Geometry check sheet. Reference: drawing and pictorial views, mm from the part's lowest x, y, z. A direction names the side the tool comes from. Coordinates: 2 decimals unless noted, no trailing zeros. Loops run counter-clockwise (first coordinate to the right, second up) from the corner with the lowest first, then second, coordinate; pieces in that order, holes last.
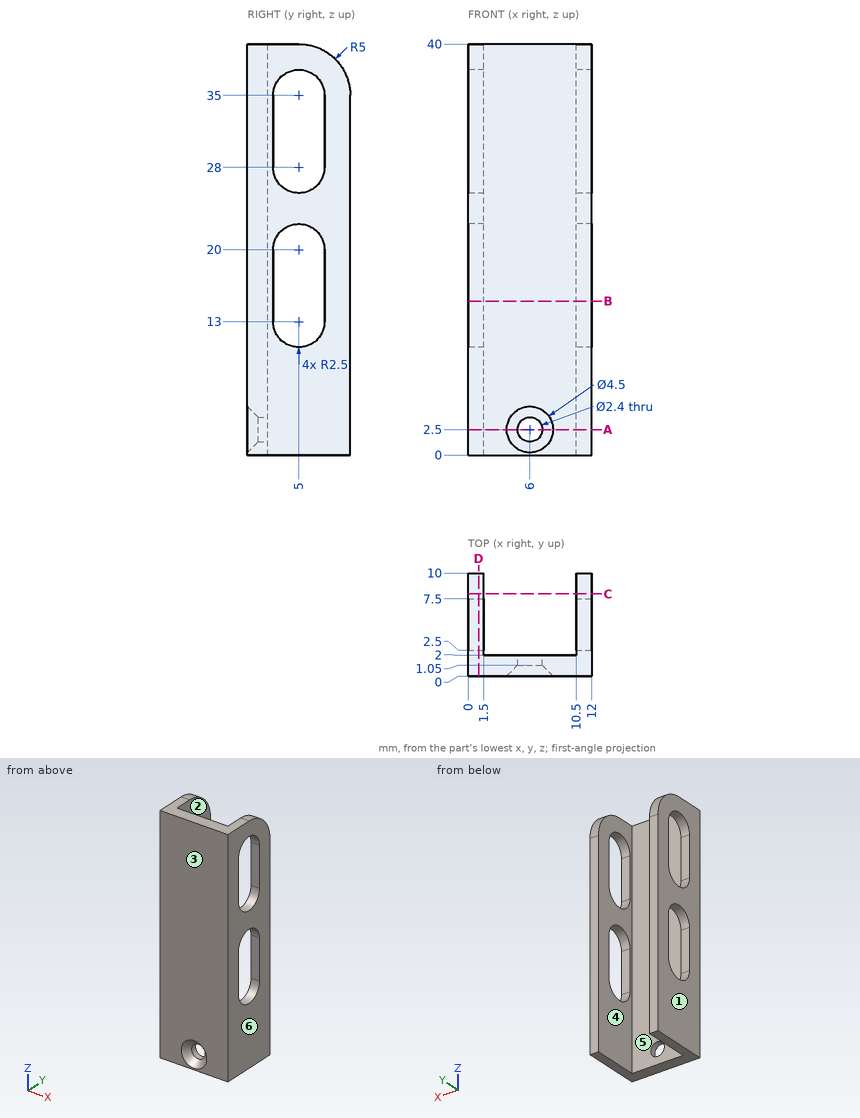
1) Depth check by flat-ended pin: pin 1 (1.2 mm diameter, centred on x = 0.5, z = 33, fed in from -Y); pin 2 (4 mm diameter, centred on x = 6, z = 2.5, fed in from +Y); pin 3 (4 mm diameter, centred on x = 8, y = 6.5, fed in from +Z). Enter the tip coordinate at first touch or a pass-through.
Data:
pin 1: stops at y = 0
pin 2: stops at y = 2
pin 3: passes through
2) Section check C-C on y = 8. Record the cut outline in (x, z).
Data:
outline: (0, 0) - (1.5, 0) - (1.5, 39) - (0, 39) - close; (10.5, 0) - (12, 0) - (12, 39) - (10.5, 39) - close
3) Section check B-B on z = 15. Record the cut outline in (x, y).
Data:
outline: (0, 0) - (12, 0) - (12, 2.5) - (10.5, 2.5) - (10.5, 2) - (1.5, 2) - (1.5, 2.5) - (0, 2.5) - close; (0, 7.5) - (1.5, 7.5) - (1.5, 10) - (0, 10) - close; (10.5, 7.5) - (12, 7.5) - (12, 10) - (10.5, 10) - close
4) Material ranges on probe 1 along X at (y, z) = (1.3, 2.5); probe 2 along Z at (x, y) = (6, 1.7); probe 3 along X at (y, z) = (8.75, 27.5), recorded low to high.
Data:
probe 1: x = 0 to 4.8, 7.2 to 12
probe 2: z = 0 to 1.3, 3.7 to 40
probe 3: x = 0 to 1.5, 10.5 to 12
5) Section check D-D on x = 1. Record the cut outline in (y, z).
Data:
outline: (0, 0) - (10, 0) - (10, 35) arc R5 ccw to (5, 40) - (0, 40) - close; hole (2.5, 13) arc R2.5 ccw to (7.5, 13) - (7.5, 20) arc R2.5 ccw to (2.5, 20) - close; hole (2.5, 28) arc R2.5 ccw to (7.5, 28) - (7.5, 35) arc R2.5 ccw to (2.5, 35) - close
6) Section check A-A on z = 2.5. Record the cut outline in (x, y), and give its area (3 significant figures).
Data:
outline: (0, 0) - (3.75, 0) - (4.8, 1.05) - (4.8, 2) - (1.5, 2) - (1.5, 10) - (0, 10) - close; (7.2, 1.05) - (8.25, 0) - (12, 0) - (12, 10) - (10.5, 10) - (10.5, 2) - (7.2, 2) - close
area: 42.1 mm2
7) Mould release check, pull along X, two halves, no side actions. Record for the marked faces 3, 4, 5 and 6: +X half, -X half, draft (parallel to the pull), parting line (faces both ways), or undercut.
Data:
face 3: draft
face 4: undercut
face 5: undercut
face 6: +X half
8) Access from +Z, -Z, +X, -X, +Y, -Y to the whole of each face (thin tool, end or side, straight path). Record for the marked faces 1 and 2.
Data:
face 1: +Z, -Z, -X, +Y, -Y
face 2: +Z, -Z, +Y
